from build123d import *

# Parameters (mm, degrees)
F0_W     = 62.165049836
F0_H     = 74.4500532746
F1_DEPTH = 25
F2_SIZE  = 5
F4_D     = 8.8
F5_R     = 5
F6_R     = 5


with BuildPart() as f1:
    # F0 (on Front) → F1 (new body)
    with BuildSketch(Plane.XZ):
        with Locations((3.1384425238, -1.9241571426)):
            Rectangle(F0_W, F0_H)
    extrude(amount=F1_DEPTH)

    # F2
    f2_edges = [f1.edges().sort_by_distance(p)[0] for p in [
        (-27.944082, 0, -1.924157),
        (3.138443, -25, 35.300869),
        (-27.944082, -25, -1.924157),
        (3.138443, -25, -39.149184),
        (34.220967, -25, -1.924157),
        (-27.944082, -12.5, 35.300869),
        (-27.944082, -12.5, -39.149184),
        (3.138443, 0, -39.149184),
        (34.220967, 0, -1.924157),
        (3.138443, 0, 35.300869),
    ]]
    chamfer(f2_edges, length=F2_SIZE)

    # F4 (through all)
    with Locations(Plane(origin=(0, 0, 0), x_dir=(-1, 0, 0), z_dir=(0, 1, 0))):
        with Locations((10.6416083872, -18.9576819539)):
            Hole(F4_D / 2)

    # F5
    f5_edges = [f1.edges().sort_by_distance(p)[0] for p in [
        (34.220967, -12.5, -39.149184),
    ]]
    fillet(f5_edges, radius=F5_R)

    # F6
    f6_edges = [f1.edges().sort_by_distance(p)[0] for p in [
        (34.220967, -12.5, 35.300869),
    ]]
    fillet(f6_edges, radius=F6_R)


solid = f1.part
Design review of the part built by this model. Coordinates are the model's own, in mm. Coordinates: 2 decimals unless noted, no trailing zeros. Order: outer loops, then holes, each group sorted by start corner. A loop starts at its lowest first (then second) coordinate and runs counter-clockwise, first axis right, second up. Notation, with made-up numbers: M 47.25,19 L 85.25,19 A16 cw 85.25,45 Z; hole C 29,-38 d1. An arc over 180 degrees is marked long. Use a Markdown table: item, result.
(1) Add section D-D (z = -17.5). Give the boundary of the cut face in (x, y).
Worked answers:
| item | result |
|---|---|
| outline | M -27.94,-20 L -22.94,-25 L -14.79,-25 L -14.79,0 L -22.94,0 L -27.94,-5 Z; M -6.49,-25 L 29.22,-25 L 34.22,-20 L 34.22,-5 L 29.22,0 L -6.49,0 Z |
(2) Draft analysis for pull direction Z (two halves, no side actions). For faces 1 (the cylindrical face through (-14.13, -12.67, -21.64)), 2 (the flat face through (31.686, -2.465, -2.425)), 3 (the flat face through (-24.45, -21.58, -36.06)), state which applies: released by +Z, released by -Z, zero draft, split by the parting line, or undercut.
Worked answers:
| item | result |
|---|---|
| face 1 | undercut |
| face 2 | zero draft |
| face 3 | released by -Z |
(3) Add section C-C (y = -8.75). Give the boundary of the cut face in (x, z).
Worked answers:
| item | result |
|---|---|
| outline | M -27.94,-34.15 L -22.94,-39.15 L 29.22,-39.15 A5 ccw 34.22,-34.15 L 34.22,30.3 A5 ccw 29.22,35.3 L -22.94,35.3 L -27.94,30.3 Z; hole C -10.64,-18.96 d8.8 |
(4) Add section A-A (z = 11.5). Give the boundary of the cut face in (x, y).
Worked answers:
| item | result |
|---|---|
| outline | M -27.94,-20 L -22.94,-25 L 29.22,-25 L 34.22,-20 L 34.22,-5 L 29.22,0 L -22.94,0 L -27.94,-5 Z |
(5) Add section B-B (x = -9). Give the boundary of the cut face in (y, z), then the cut area to 3 significant figures.
Worked answers:
| item | result |
|---|---|
| outline | M -25,-34.15 L -20,-39.15 L -5,-39.15 L 0,-34.15 L 0,-23.04 L -25,-23.04 Z; M -25,-14.88 L 0,-14.88 L 0,30.3 L -5,35.3 L -20,35.3 L -25,30.3 Z |
| area | 1,610 mm2 |
(6) Wall thickness on probe 1 along X at (y, z) = (-10.75, -21); probe 2 along Z at (x, y) = (18.5, -22.25); probe 3 along Z at (x, y) = (-7, -22): over which ranges is each line inside the solid? List them lowest first.
Worked answers:
| item | result |
|---|---|
| probe 1 | x = -27.94 to -14.54, -6.74 to 34.22 |
| probe 2 | z = -36.9 to 33.05 |
| probe 3 | z = -37.15 to -21.43, -16.49 to 33.3 |
(7) For P1, Ø6, axis at x = -12, z = -21, coming from the +Y side; P2, Ø2, axis at x = -5.5, y = -3, coming from the +Z side, all flat-tipped, find the tip position at first contact; note any pin that passes through.
Worked answers:
| item | result |
|---|---|
| P1 | stops at y = 0 |
| P2 | stops at z = 34.3 |
